from build123d import *

# Parameters (mm, degrees)
F1_DEPTH = 12.7
F2_W     = 171.45
F2_H     = 103.8304664585
F3_DEPTH = 25.4
F4_DEPTH = 25.4
F5_W     = 38.1
F5_H     = 6.35
F6_DEPTH = 12.7


with BuildPart() as f1:
    # F0 (on Top) → F1 (new body)
    with BuildSketch(Plane.XY):
        with BuildLine():
            Line((65.9010224927, -54.4816457485), (65.9010224927, -29.0816457485))
            Line((65.9010224927, -29.0816457485), (78.6010224927, -29.0816457485))
            Line((78.6010224927, -29.0816457485), (78.6010224927, 15.3683542515))
            ThreePointArc((78.6010224927, 15.3683542515), (-0.3807983971, 36.6148097647), (-80.1489775073, 18.5433542515))
            Line((-80.1489775073, 18.5433542515), (-80.1489775073, -16.3816457485))
            Line((-80.1489775073, -16.3816457485), (27.8010224927, -16.3816457485))
            Line((27.8010224927, -16.3816457485), (27.8010224927, -54.4816457485))
            Line((27.8010224927, -54.4816457485), (65.9010224927, -54.4816457485))
        make_face()
    extrude(amount=F1_DEPTH)

    # F2 (on face) → F3 (join)
    with BuildSketch(Plane(origin=(0, 0, 0), x_dir=(1, 0, 0), z_dir=(0, 0, -1))):
        with Locations((-0.7739775073, 8.9164125192)):
            Rectangle(F2_W, F2_H)
    extrude(amount=F3_DEPTH)

    # F4 (cut): a face of the model
    f4_faces = [f1.faces().sort_by_distance(p)[0] for p in [
        (7.501284612, -0.1265709207, 12.7),
    ]]
    extrude(f4_faces, amount=-F4_DEPTH, mode=Mode.SUBTRACT)

    # F5 (on face) → F6 (cut)
    with BuildSketch(Plane.XY):
        with Locations((46.8510224927, -57.6566457485)):
            Rectangle(F5_W, F5_H)
    extrude(amount=-F6_DEPTH, mode=Mode.SUBTRACT)


solid = f1.part
Check sheet for the modelled part. Datum: model origin and axes. Units: mm. A direction names the side the tool comes from. Give positions to 0.01 mm unless a question says otherwise; leave off trailing zeros. Write each loop counter-clockwise with the first axis right and the second up, starting at its lowest first coordinate (ties: lowest second). Pieces come first, ordered by that corner, then holes. Notation, with made-up numbers: M 73.25,12 L 129.25,12 A30 cw 129.25,48 Z; hole C 33.5,23.25 d7. An arc over 180 degrees is marked long. Use one line per item in the form item = value.
(1) Section check B-B on x = 13. Record the boundary of the cut face in (y, z), plus the area to 3 significant figures.
Answer block:
outline = M -60.83,-25.4 L 43,-25.4 L 43,0 L 35.82,0 L 35.82,-12.7 L -16.38,-12.7 L -16.38,0 L -60.83,0 Z
area = 1,970 mm2
(2) Section check A-A on z = -6.75. Record the boundary of the cut face in (x, y), plus the area to 3 significant figures.
Answer block:
outline = M -86.5,-60.83 L 27.8,-60.83 L 27.8,-16.38 L -80.15,-16.38 L -80.15,18.54 A170.11 cw 78.6,15.37 L 78.6,-29.08 L 65.9,-29.08 L 65.9,-60.83 L 84.95,-60.83 L 84.95,43 L -86.5,43 Z
area = 8,550 mm2
(3) Section check D-D on x = 31. Record the boundary of the cut face in (y, z).
Answer block:
outline = M -60.83,-25.4 L 43,-25.4 L 43,0 L 33.05,0 L 33.05,-12.7 L -60.83,-12.7 Z
(4) Tool access check on faces 5 (the flat face through (65.901, -45, -6)), 6 (the flat face through (-2, -10, -25.4)), 7 (the cylindrical face through (0.775, 36.588, -6.261)). Record the directions out of +Z, -Z, +X, -X, +Y, -Y that give a thin tool (end or side, any length) a straight path to the whole face; none if there is none.
Answer block:
face_5 = +Z, -Y
face_6 = -Z, +X, -X, +Y, -Y
face_7 = +Z
(5) Draft check along X on faces 1 (the flat face through (-86.499, -8, -13)), 2 (the flat face through (84.951, -8, -13)), 3 (the flat face through (78.601, -7, -6)), 4 (the flat face through (-2, 42.999, -13)). Enter one of: pulls with the +X half, pulls with the -X half, needs draft (parallel to the pull), parting line crosses it, or undercut.
Answer block:
face_1 = pulls with the -X half
face_2 = pulls with the +X half
face_3 = undercut
face_4 = needs draft
(6) Material ranges on line 1 along X through (y, z) = (9, -10); line 2 along Z through (x, y) = (43, -27); line 3 along X through (y, z) = (-51, -2.25), recorded low to high.
Answer block:
line_1 = -86.5 to -80.15, 78.6 to 84.95
line_2 = -25.4 to -12.7
line_3 = -86.5 to 27.8, 65.9 to 84.95
(7) Depth check by flat-ended pin: P1, Ø8, axis at x = 42.5, y = 20.5, coming from the +Z side. Enter the tip coordinate at first touch or a pass-through.
Answer block:
P1 = -12.7
(8) Section check C-C on y = 2.5. Record the boundary of the cut face in (x, z).
Answer block:
outline = M -86.5,-25.4 L 84.95,-25.4 L 84.95,0 L 78.6,0 L 78.6,-12.7 L -80.15,-12.7 L -80.15,0 L -86.5,0 Z
